Design review of the part built by this model. Coordinates are the model's own, in mm. Face numbers are marked on the shaded views. Give positions to 0.01 mm unless a question says otherwise; leave off trailing zeros. Loops run counter-clockwise (first coordinate to the right, second up) from the corner with the lowest first, then second, coordinate; pieces in that order, holes last. Notation, with made-up numbers: M -8,41.25 L 40,41.25 A25 ccw 40,56.25 Z; hole C -4.5,20.5 d10. An arc over 180 degrees is marked long. Use CSV: the item, a comma, the result in double quotes.
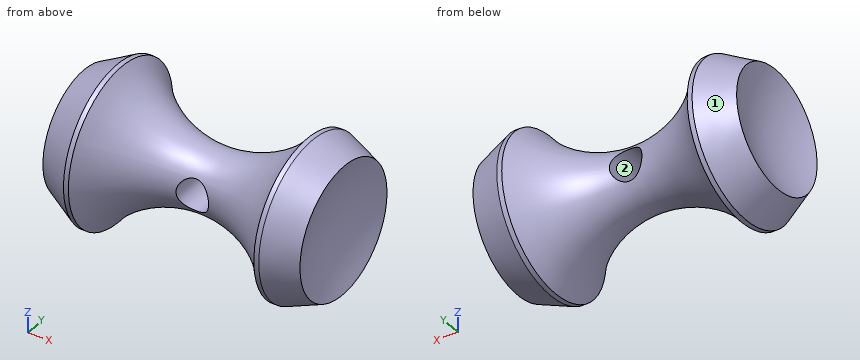
Autodesk Inventor part; units mm, degrees
ref_plane "YZ Plane" through (0, 0, 0) normal (1, 0, 0) x (0, 1, 0)
ref_plane "XZ Plane" through (0, 0, 0) normal (0, 1, 0) x (-1, 0, 0)
ref_plane "XY Plane" through (0, 0, 0) normal (0, 0, 1) x (1, 0, 0)
sketch "草圖1" plane through (0, 0, 0) normal (0, 0, 1) x (1, 0, 0)
  line L0 (0, 18.5) -> (10, 24)
  line L1 (10, 24) -> (11.5, 24)
  line L2 (80, 20) -> (70, 24)
  line L3 (70, 24) -> (68.5, 24)
  line L4 (0, 0) -> (80, 0)
  arc A0 (11.5, 24) -> (68.5, 24) centre (40, 44.3162) ccw
  arc A1 (4.5352, 0) -> (0, 18.5) centre (-35.4648, 0) ccw
  arc A2 (80, 20) -> (75.8258, 0) centre (125.8258, 0) ccw
  dimension "d0" = 18.5
  dimension "d2" = 1.5
  dimension "d3" = 1.5
  dimension "d4" = 24
  dimension "d6" = 20
  dimension "d8" = 24
  dimension "d9" = 35
  dimension "d21" = 40
  dimension "d23" = 50
  dimension "d33" = 158.199
  dimension "d34" = 129.388
  dimension "d35" = 48.2808
  dimension "d36" = 16.21
  dimension "d37" = 1.5503
  dimension "d38" = 24
  dimension "d39" = 46.5964
revolve "迴轉1" add sketch "草圖1" angle 360 about axis through (0, 0, 0) along (1, 0, 0)
sketch "草圖2" plane through (0, 0, 0) normal (0, 1, 0) x (-1, 0, 0)
  circle A0 centre (-40, 0) radius 5
  point P0 (0, 0)
  dimension "d11" = 10
  dimension "d12" = 0
  dimension "d13" = 40
extrude "擠出1" cut sketch "草圖2" along normal mid plane 60
properties part number "A"
(1) We need section A-A on x = 40. State the section outline as (y, z) points.
A:
outline,"M -7.86,-5 A9.32 ccw 7.86,-5 Z; M -7.86,5 L 7.86,5 A9.32 ccw Z"
(2) Wall thickness on line 1 along X through (y, z) = (14.5, -8.5); line 2 along Z through (x, y) = (40, 0); line 3 along X through (y, z) = (6, -21.5): over which ranges is each line inside the solid? List them lowest first. Write a range as [from, to].
A:
line 1,"[0.83, 18.36], [61.64, 78.74]"
line 2,"[-9.32, -5], [5, 9.32]"
line 3,"[6.95, 12.77], [67.23, 74.2]"
(3) We need section B-B on x = 71. State the section outline as (y, z) points, then the cut area to 3 significant figures.
A:
outline,"C 0,0 d47.2"
area,"1,750 mm²"
(4) The part is to be moulded in two halves that separate along Z. For the marked faces 1 and 2, say which applies: released by +Z, released by -Z, zero draft, split by the parting line, or undercut.
A:
face 1,"split by the parting line"
face 2,"undercut"
(5) We need section C-C on x = 25. State the section outline as (y, z) points.
A:
outline,"C 0,0 d25.39"
(6) Clearance check with flat-ended pins moving along their axes: P1, Ø3, axis at y = 6.5, z = 11, coming from the -X side; P2, Ø4, axis at y = -11.5, z = 2.5, coming from the +X side; P3, Ø1.5, axis at x = 57.5, z = 1, coming from the -Y side. State where each tip first meets the part, or that it passes through.
A:
P1,"x = 1.9"
P2,"x = 77.76"
P3,"y = -14.42"
